from build123d import *

# Parameters (mm, degrees)
CHAMFER_SIZE = 0.4
FILLET_R     = 0.2
POCKET_DEPTH = 2


with BuildPart() as part:
    # Sketch → Revolution (revolve)
    with BuildSketch(Plane.XZ):
        Polygon((2, 0), (2, 10), (3.5, 10), (3.5, 14), (0, 14), (0, 0), align=None)
    revolve(axis=Axis((0, 0, 0), (0, 0, 1)))

    # Chamfer
    chamfer_edges = [part.edges().sort_by_distance(p)[0] for p in [
        (-2, 0, 0),
    ]]
    chamfer(chamfer_edges, length=CHAMFER_SIZE)

    # Fillet
    fillet_edges = [part.edges().sort_by_distance(p)[0] for p in [
        (-3.5, 0, 14),
    ]]
    fillet(fillet_edges, radius=FILLET_R)

    # Sketch001 (on Face6 of Chamfer) → Pocket (cut)
    with BuildSketch(Plane(origin=(0, 0, 14), x_dir=(-1, 0, 0), z_dir=(0, 0, 1))):
        Polygon((1.5, 0.866025), (0, 1.732051), (-1.5, 0.866025), (-1.5, -0.866025), (0, -1.732051), (1.5, -0.866025), align=None)
    extrude(amount=-POCKET_DEPTH, mode=Mode.SUBTRACT)


solid = part.part
Verification items for the finished model (mm, model axes). A direction names the side the tool comes from. Give positions to 0.01 mm unless a question says otherwise; leave off trailing zeros. Order: outer loops, then holes, each group sorted by start corner. A loop starts at its lowest first (then second) coordinate and runs counter-clockwise, first axis right, second up. Notation, with made-up numbers: M -37.5,7.5 L -1.5,7.5 A25 ccw -1.5,35.5 Z; hole C -31.75,75.25 d2. An arc over 180 degrees is marked long. Answer as a JSON object with one key per item and string values. Group by question number.
1) Cross-section at A-A (y = 0). Enter the section's corners in (x, z), then the cut area to 3 significant figures.
2) Depth check by flat-ended pin: pin 1 Ø1.5 at (x, z) = (2, 6) entering from +Y; pin 2 Ø1.5 at (x, z) = (2.5, 6) entering from -Y; pin 3 Ø1.5 at (y, z) = (-2.5, 3) entering from -X. Enter the tip coordinate at first touch or a pass-through.
3) Mould release check, pull along X, two halves, no side actions. Record for faces 1 (the face through (-2, 0, 14)), 2 (the face through (0, -2, 5)), 3 (the face through (-0.74, 1.305, 13.014)): released by +X, released by -X, zero draft, split by the parting line, or undercut.
4) Access from +Z, -Z, +X, -X, +Y, -Y to the whole of each face (thin tool, end or side, straight path). Record for faces 4 (the face through (0, 0, 0)), 5 (the face through (-2, -2, 10)), 6 (the face through (0, 0, 12)).
5) Scan lines: line 1 along Z through (x, y) = (2.75, -0.5); line 2 along Z through (x, y) = (1, -0.5); line 3 along X through (y, z) = (-1, 8.5). Record each from-to range of solid material in increasing order. Write a range as [from, to].
6) Cross-section at C-C (z = 2). Enter the section's corners in (x, y).
7) Cross-section at B-B (z = 11.5). Enter the section's corners in (x, y).
Result sheet:
{
 "1": {"outline": "M -3.5,10 L -2,10 L -2,0.4 L -1.6,0 L 1.6,0 L 2,0.4 L 2,10 L 3.5,10 L 3.5,13.8 A0.2 ccw 3.3,14 L 1.5,14 L 1.5,12 L -1.5,12 L -1.5,14 L -3.3,14 A0.2 ccw -3.5,13.8 Z", "area": "61.8 mm2"},
 "2": {"pin 1": "stops at y = 1.56", "pin 2": "stops at y = -0.97", "pin 3": "stops at x = -0.97"},
 "3": {"face 1": "zero draft", "face 2": "split by the parting line", "face 3": "undercut"},
 "4": {"face 4": "-Z, +X, -X, +Y, -Y", "face 5": "-Z", "face 6": "+Z"},
 "5": {"line 1": "z = [10, 14]", "line 2": "z = [0, 12]", "line 3": "x = [-1.73, 1.73]"},
 "6": {"outline": "C 0,0 d4"},
 "7": {"outline": "C 0,0 d7"}
}
